The listing builds one solid part. Answer for the finished solid, in the listing's coordinates (mm). Face numbers are marked on the shaded views. A direction names the side the tool comes from. Coordinates: 2 decimals unless noted, no trailing zeros. Loops run counter-clockwise (first coordinate to the right, second up) from the corner with the lowest first, then second, coordinate; pieces in that order, holes last. Notation, with made-up numbers: (4.5, -24.75) - (50.5, -24.75) arc R4 ccw to (50.5, -17.75) - close; hole circle Ø2 at (-14, 78). An arc over 180 degrees is marked (long way). Put each result on its own line as item: value.
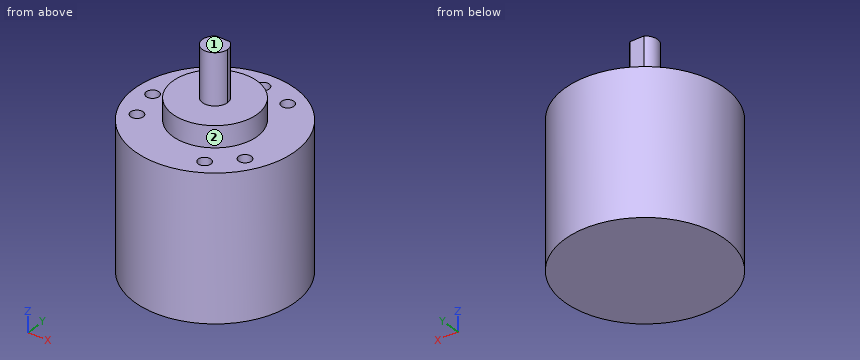
```python
from build123d import *

# Parameters (mm, degrees)
SKETCH1_R           = 19
BOSS_EXTRUDE1_DEPTH = 34
SKETCH2_R           = 1.5
CUT_EXTRUDE1_DEPTH  = 6
SKETCH3_R           = 10
BOSS_EXTRUDE2_DEPTH = 5
BOSS_EXTRUDE3_DEPTH = 12


with BuildPart() as part:
    # Sketch1 → Boss-Extrude1 (new body)
    with BuildSketch(Plane.XY):
        Circle(SKETCH1_R)
    extrude(amount=BOSS_EXTRUDE1_DEPTH)

    # Sketch2 → Cut-Extrude1 (cut)
    with BuildSketch(Plane.XY.offset(34)):
        with Locations((-12.990381057, -7.5)):
            Circle(SKETCH2_R)
        with Locations((-15, 0)):
            Circle(SKETCH2_R)
        with Locations((0, 15)):
            Circle(SKETCH2_R)
        with Locations((7.5, 12.990381057)):
            Circle(SKETCH2_R)
        with Locations((12.990381057, -7.5)):
            Circle(SKETCH2_R)
        with Locations((7.5, -12.990381057)):
            Circle(SKETCH2_R)
    extrude(amount=-CUT_EXTRUDE1_DEPTH, mode=Mode.SUBTRACT)

    # Sketch3 → Boss-Extrude2 (add)
    with BuildSketch(Plane.XY.offset(34)):
        Circle(SKETCH3_R)
    extrude(amount=BOSS_EXTRUDE2_DEPTH)

    # Sketch4 → Boss-Extrude3 (add)
    with BuildSketch(Plane.XY.offset(39)):
        with BuildLine():
            ThreePointArc((3, 0), (2.643382037, 1.418637165), (1.658312395, 2.5))
            Line((1.658312395, 2.5), (-1.658312395, 2.5))
            ThreePointArc((-1.658312395, 2.5), (-1.418637165, -2.643382037), (3, 0))
        make_face()
    extrude(amount=BOSS_EXTRUDE3_DEPTH)


solid = part.part
```
1) The part is cut by section A-A (x = 0). Give the vertices of the cut face in (y, z).
Found:
outline: (-19, 0) - (19, 0) - (19, 34) - (16.5, 34) - (16.5, 28) - (13.5, 28) - (13.5, 34) - (10, 34) - (10, 39) - (2.5, 39) - (2.5, 51) - (-3, 51) - (-3, 39) - (-10, 39) - (-10, 34) - (-19, 34) - close
2) For the marked faces 1 and 2, determine the directions among +Z, -Z, +X, -X, +Y, -Y from which every point of the face is accessible in a straight line to the end or side of a thin tool.
Found:
face 1: +Z, +X, -X, +Y, -Y
face 2: +Z
3) Each of these flat-tipped pins is pushed along its axis until it touches: pin 1 (1 mm diameter, centred on x = 0.5, z = 43.5, fed in from +Y); pin 2 (12 mm diameter, centred on y = -15, z = 25.5, fed in from -X); pin 3 (2.5 mm diameter, centred on x = -0.5, y = 15, fed in from +Z). Where does it stop, or does it pass through?
Found:
pin 1: stops at y = 2.5
pin 2: stops at x = -16.73
pin 3: stops at z = 34
4) The part is cut by section B-B (y = -7.5). Give the vertices of the cut face in (x, z).
Found:
outline: (-17.46, 0) - (17.46, 0) - (17.46, 34) - (14.49, 34) - (14.49, 28) - (11.49, 28) - (11.49, 34) - (6.61, 34) - (6.61, 39) - (-6.61, 39) - (-6.61, 34) - (-11.49, 34) - (-11.49, 28) - (-14.49, 28) - (-14.49, 34) - (-17.46, 34) - close
5) The part is cut by section C-C (z = 29). Give the vertices of the cut face in (x, y).
Found:
outline: circle Ø38 at (0, 0); hole circle Ø3 at (-15, 0); hole circle Ø3 at (-12.99, -7.5); hole circle Ø3 at (0, 15); hole circle Ø3 at (7.5, -12.99); hole circle Ø3 at (7.5, 12.99); hole circle Ø3 at (12.99, -7.5)
6) Straight lines are drawn through the part: L1, parallel to Y at x = 0, z = 30; L2, parallel to Z at x = -16, y = 4.5; L3, parallel to Z at x = -8.5, y = -4. For each, find the intervals that lie inside material, in ascending order. Write a range as [from, to].
Found:
L1: y = [-19, 13.5], [16.5, 19]
L2: z = [0, 34]
L3: z = [0, 39]
7) The part is cut by section D-D (z = 46.5). Give the vertices of the cut face in (x, y).
Found:
outline: (-1.66, 2.5) arc R3 ccw (long way) to (1.66, 2.5) - close
